Drawing for the job (mm, zero at the part's lowest x, y, z). Coordinates: 2 decimals unless noted, no trailing zeros. Order: outer loops, then holes, each group sorted by start corner. A loop starts at its lowest first (then second) coordinate and runs counter-clockwise, first axis right, second up.
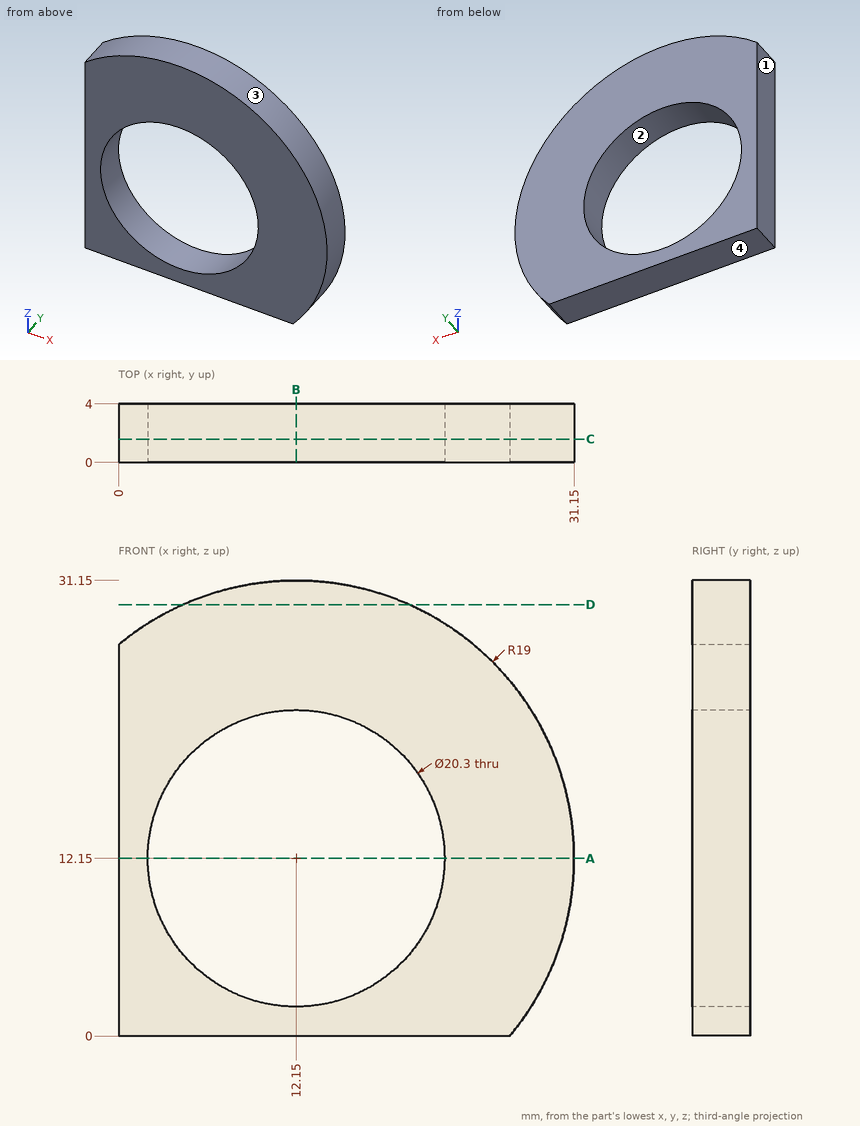
(1) Slice it at C-C, the plane y = 1.6. Give the cut face in (x, z), then the cut area to 3 significant figures.
(2) Slice it at A-A, the plane z = 12.15. Give the cut face in (x, y), then the cut area to 3 significant figures.
(3) Probe line 1 (X direction, y = 1.25, z = 12.15); line 2 (Z direction, x = 3.5, y = 0.7); line 3 (X direction, y = 3.1, z = 9). List the from-to ranges inside material, lowest first.
(4) Slice it at B-B, the plane x = 12.15. Give the cut face in (y, z), then the cut area to 3 significant figures.
(5) Slice it at D-D, the plane z = 29.5. Give the cut face in (x, y), then the cut area to 3 significant figures.
(6) Drop a flat-ended pin along its axis: pin 1 (1 mm diameter, centred on x = 27.5, y = 1, fed in from +Z). Give the stop position or say it passes through.
(7) Pull direction X, two halves, no side cores. Call the marked faces 1, 2, 3 and 4: +X half, -X half, draft (parallel to the pull), parting line (faces both ways), or undercut.
Here are the results:
1. outline: (0, 0) - (26.76, 0) arc R19 ccw to (0, 26.76) - close; hole circle Ø20.3 at (12.15, 12.15)
1. area: 535 mm2
2. outline: (0, 0) - (2, 0) - (2, 4) - (0, 4) - close; (22.3, 0) - (31.15, 0) - (31.15, 4) - (22.3, 4) - close
2. area: 43.4 mm2
3. line 1: x = 0 to 2, 22.3 to 31.15
3. line 2: z = 0 to 6.84, 17.46 to 29.07
3. line 3: x = 0 to 2.5, 21.8 to 30.89
4. outline: (0, 0) - (4, 0) - (4, 2) - (0, 2) - close; (0, 22.3) - (4, 22.3) - (4, 31.15) - (0, 31.15) - close
4. area: 43.4 mm2
5. outline: (4.41, 0) - (19.89, 0) - (19.89, 4) - (4.41, 4) - close
5. area: 62.0 mm2
6. pin 1: stops at z = 24
7. face 1: -X half
7. face 2: undercut
7. face 3: parting line
7. face 4: draft
